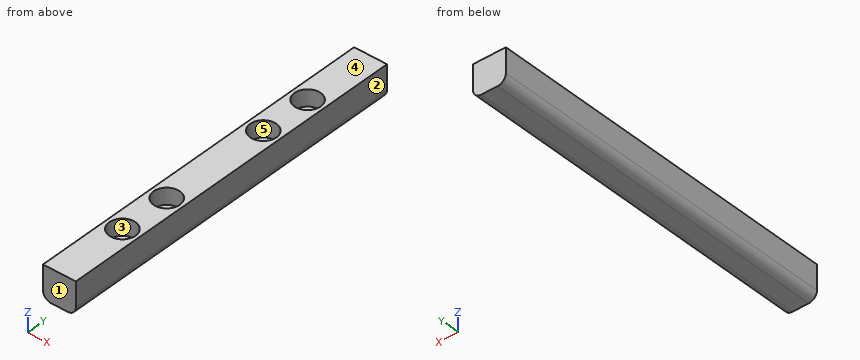
```python
from build123d import *

# Parameters (mm, degrees)
SKETCH2_W           = 10
SKETCH2_H           = 110
BOSS_EXTRUDE1_DEPTH = 10
SKETCH3_R           = 4
CUT_EXTRUDE1_DEPTH  = 5
FILLET1_R           = 2.5


with BuildPart() as part:
    # Sketch2 → Boss-Extrude1 (new body)
    with BuildSketch(Plane.XY):
        with Locations((5, 55)):
            Rectangle(SKETCH2_W, SKETCH2_H)
    extrude(amount=BOSS_EXTRUDE1_DEPTH)

    # Sketch3 → Cut-Extrude1 (cut)
    with BuildSketch(Plane.XY.offset(10)):
        with Locations((5, 87.731895651)):
            Circle(SKETCH3_R)
        with Locations((5, 72.077510774)):
            Circle(SKETCH3_R)
        with Locations(Location((5, 37.922489226, 0), (0, 0, 180))):
            Circle(SKETCH3_R)
        with Locations(Location((5, 22.268104349, 0), (0, 0, 180))):
            Circle(SKETCH3_R)
    extrude(amount=-CUT_EXTRUDE1_DEPTH, mode=Mode.SUBTRACT)

    # Fillet1
    fillet1_edges = [part.edges().sort_by_distance(p)[0] for p in [
        (0, 55, 0),
        (10, 55, 0),
    ]]
    fillet(fillet1_edges, radius=FILLET1_R)


solid = part.part
```
Check sheet for the modelled part. Datum: model origin and axes. Units: mm. Face numbers are marked on the shaded views. A direction names the side the tool comes from. Give positions to 0.01 mm unless a question says otherwise; leave off trailing zeros. Write each loop counter-clockwise with the first axis right and the second up, starting at its lowest first coordinate (ties: lowest second). Pieces come first, ordered by that corner, then holes. Notation, with made-up numbers: (33, -23) -> (44, -23) arc R7 ccw to (44, -11) -> close; hole circle Ø3 at (52.25, 77). An arc over 180 degrees is marked (long way). Use CSV: the item, a comma, the result in double quotes. Start each with the question number.
Q1. Cross-section at B-B on z = 8.25. Enter the section's corners in (x, y).
Q2. Scan lines: line 1 along Y through (x, z) = (5, 8.55); line 2 along Y through (x, z) = (8.25, 6.75); line 3 along Z through (x, y) = (0.5, 47). Record each from-to range of solid material in increasing order.
Q3. Tool access check on the marked faces 4 and 5. Record the directions out of +Z, -Z, +X, -X, +Y, -Y that give a thin tool (end or side, any length) a straight path to the whole face; none if there is none.
Q4. Cross-section at D-D on z = 1.25. Enter the section's corners in (x, y).
Q5. Cross-section at C-C on x = 5. Enter the section's corners in (y, z).
Q6. Release check for a two-part mould opening along Y. For the marked faces 1, 2 and 3 record: +Y half, -Y half, draft (parallel to the pull), parting line (faces both ways), or undercut.
Q7. Cross-section at A-A on y = 95.5. Enter the section's corners in (x, z), and give its area (3 significant figures).
Working result:
1,outline,"(0, 0) -> (10, 0) -> (10, 110) -> (0, 110) -> close; hole circle Ø8 at (5, 22.27); hole circle Ø8 at (5, 37.92); hole circle Ø8 at (5, 72.08); hole circle Ø8 at (5, 87.73)"
2,line 1,"y = 0 to 18.27, 26.27 to 33.92, 41.92 to 68.08, 76.08 to 83.73, 91.73 to 110"
2,line 2,"y = 0 to 19.94, 24.6 to 35.59, 40.25 to 69.75, 74.41 to 85.4, 90.06 to 110"
2,line 3,"z = 1 to 10"
3,face 4,"+Z, +X, -X, +Y, -Y"
3,face 5,"+Z"
4,outline,"(0.33, 0) -> (9.67, 0) -> (9.67, 110) -> (0.33, 110) -> close"
5,outline,"(0, 0) -> (110, 0) -> (110, 10) -> (91.73, 10) -> (91.73, 5) -> (83.73, 5) -> (83.73, 10) -> (76.08, 10) -> (76.08, 5) -> (68.08, 5) -> (68.08, 10) -> (41.92, 10) -> (41.92, 5) -> (33.92, 5) -> (33.92, 10) -> (26.27, 10) -> (26.27, 5) -> (18.27, 5) -> (18.27, 10) -> (0, 10) -> close"
6,face 1,"-Y half"
6,face 2,"draft"
6,face 3,"undercut"
7,outline,"(0, 2.5) arc R2.5 ccw to (2.5, 0) -> (7.5, 0) arc R2.5 ccw to (10, 2.5) -> (10, 10) -> (0, 10) -> close"
7,area,"97.3 mm^2"
